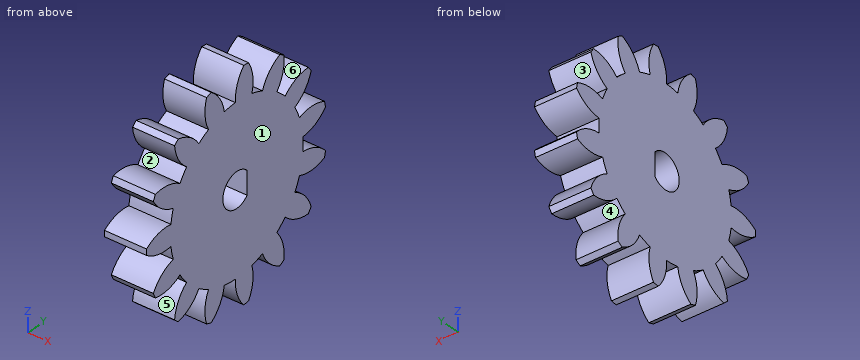
```python
from build123d import *

# Parameters (mm, degrees)
BASPROSKE_W        = 6.35
BASPROSKE_H        = 17
TOOTHCUT_DEPTH     = 25.86609137
TEETHCUTS_COUNT    = 15
BORSKE_R           = 0.4
BORE_DEPTH         = 50.0000508
CUT_EXTRUDE1_REACH = 26.831


with BuildPart() as part:
    # BasProSke → Base-Revolve (revolve)
    with BuildSketch(Plane(origin=(0, 0, 0), x_dir=(1, 0, 0), z_dir=(0, 1, 0)), mode=Mode.PRIVATE) as base_revolve_sk:
        with Locations((3.175, 8.5)):
            Rectangle(BASPROSKE_W, BASPROSKE_H)
    revolve(base_revolve_sk.sketch.rotate(Axis((-10, 0, 0), (1, 0, 0)), 180), axis=Axis((-10, 0, 0), (1, 0, 0)))

    # TooCutSke → ToothCut (cut, through all)
    with BuildSketch(Plane(origin=(0, 0, 0), x_dir=(0, 0, -1), z_dir=(1, 0, 0))):
        with BuildLine():
            ThreePointArc((1.050056448, 12.454813626), (0, 12.499), (-1.050056448, 12.454813626))
            ThreePointArc((-1.050056448, 12.454813626), (-1.638118106, 14.809604533), (-3.110934279, 16.73876737))
            ThreePointArc((-3.110934279, 16.73876737), (0, 17.0254), (3.110934279, 16.73876737))
            ThreePointArc((3.110934279, 16.73876737), (1.638118106, 14.809604533), (1.050056448, 12.454813626))
        make_face()
    toothcut = extrude(amount=TOOTHCUT_DEPTH, mode=Mode.SUBTRACT)

    # TeethCuts: ToothCut ×15 about axis
    teethcuts_axis = Axis((0, 0, 0), (1, 0, 0))
    for i in range(1, TEETHCUTS_COUNT):
        add(toothcut.rotate(teethcuts_axis, i * 360 / TEETHCUTS_COUNT), mode=Mode.SUBTRACT)

    # BorSke → Bore (cut, symmetric)
    with BuildSketch(Plane(origin=(0, 0, 0), x_dir=(0, 0, -1), z_dir=(1, 0, 0))):
        with Locations(Location((0, 0, 0), (0, 0, 180))):
            Circle(BORSKE_R)
    extrude(amount=BORE_DEPTH, both=True, mode=Mode.SUBTRACT)

    # Sketch1 → Cut-Extrude1 (cut, up to next)
    with BuildSketch(Plane.ZY, mode=Mode.PRIVATE) as cut_extrude1_sk1:
        with BuildLine():
            Line((1.659895813, 1.69164), (-1.659895813, 1.69164))
            ThreePointArc((-1.659895813, 1.69164), (-0.917318626, -2.185274934), (2.37, 0))
            ThreePointArc((2.37, 0), (2.185274934, 0.917318626), (1.659895813, 1.69164))
        make_face()
    cut_extrude1_tool1 = extrude(cut_extrude1_sk1.sketch, amount=-CUT_EXTRUDE1_REACH, mode=Mode.PRIVATE) & part.part
    # Sketch1 → Cut-Extrude1 (cut, up to next)
    with BuildSketch(Plane.ZY, mode=Mode.PRIVATE) as cut_extrude1_sk2:
        with BuildLine():
            ThreePointArc((-1.75910037, 1.94164), (0, -2.62), (1.75910037, 1.94164))
            Line((1.75910037, 1.94164), (-1.75910037, 1.94164))
        make_face()
    cut_extrude1_tool2 = extrude(cut_extrude1_sk2.sketch, amount=-CUT_EXTRUDE1_REACH, mode=Mode.PRIVATE) & part.part
    add(cut_extrude1_tool1.solids().sort_by_distance((0, -0.189427, 0))[0], mode=Mode.SUBTRACT)
    add(cut_extrude1_tool2.solids().sort_by_distance((0, -0.182106, 0))[0], mode=Mode.SUBTRACT)


solid = part.part
```
Source: CAD feature listing. Evaluate the final solid. Frame: model axes, mm. Face numbers are marked on the shaded views. A direction names the side the tool comes from. Round coordinates to 2 decimals unless told otherwise and drop trailing zeros. Loops run counter-clockwise (first coordinate to the right, second up) from the corner with the lowest first, then second, coordinate; pieces in that order, holes last.
1. Section query C-C on z = 9. Output: boundary loops of the cut face in (x, y), and give its area (3 significant figures).
2. Ray query, L1, parallel to Y at x = 3.5, z = 0; L2, parallel to Z at x = 3.25, y = -10.5; L3, parallel to Z at x = 1, y = 0.5. Return the intervals inside material, ascending.
3. Mould query, pull axis Y, two halves, no side actions, for the marked faces 1, 2 and 3. Classes: released by +Y, released by -Y, zero draft, split by the parting line, or undercut.
4. Section query B-B on y = -13.5. Output: boundary loops of the cut face in (x, z).
5. Section query A-A on z = 0. Output: boundary loops of the cut face in (x, y), and give its area (3 significant figures).
6. Contact query for flat-ended pins moving along their axis: pin 1 (2 mm diameter, centred on y = 5, z = 5.5, fed in from -X); pin 2 (3 mm diameter, centred on y = 0, z = 0, fed in from +X); pin 3 (1.5 mm diameter, centred on x = 5.5, z = 12, fed in from +Y). Output: stop coordinate, or through.
7. Section query D-D on y = 8.5. Output: boundary loops of the cut face in (x, z).
8. Access query for the marked faces 4, 5 and 6. Directions: +Z, -Z, +X, -X, +Y, -Y. A direction counts if a zero-diameter tool reaches every point of the face in a straight line with its end or side. Return the directions, or none.
Answers below:
1. outline: (0, -10.32) - (6.35, -10.32) - (6.35, 8.67) - (0, 8.67) - close; (0, 9.6) - (6.35, 9.6) - (6.35, 13.79) - (0, 13.79) - close
1. area: 147 mm2
2. L1: y = -17 to -2.62, 1.94 to 12.5
2. L2: z = -12.8 to -9.23, -6.78 to 6.78, 9.23 to 12.8
2. L3: z = -15.82 to -2.57, 2.57 to 15.82
3. face 1: zero draft
3. face 2: undercut
3. face 3: released by +Y
4. outline: (0, -7.45) - (6.35, -7.45) - (6.35, -4.25) - (0, -4.25) - close; (0, -1.65) - (6.35, -1.65) - (6.35, 1.65) - (0, 1.65) - close; (0, 4.25) - (6.35, 4.25) - (6.35, 7.45) - (0, 7.45) - close
5. outline: (0, -17) - (6.35, -17) - (6.35, -2.62) - (0, -2.62) - close; (0, 1.94) - (6.35, 1.94) - (6.35, 12.5) - (0, 12.5) - close
5. area: 158 mm2
6. pin 1: stops at x = 0
6. pin 2: passes through
6. pin 3: stops at y = 8.84
7. outline: (0, -14.72) - (6.35, -14.72) - (6.35, -11.55) - (0, -11.55) - close; (0, -9.16) - (6.35, -9.16) - (6.35, 9.16) - (0, 9.16) - close; (0, 11.55) - (6.35, 11.55) - (6.35, 14.72) - (0, 14.72) - close
8. face 4: +X, -X
8. face 5: +X, -X, -Y
8. face 6: +Z, +X, -X
